Check sheet for the modelled part. Datum: model origin and axes. Units: mm. A direction names the side the tool comes from. Round coordinates to 2 decimals unless told otherwise and drop trailing zeros. Order: outer loops, then holes, each group sorted by start corner. A loop starts at its lowest first (then second) coordinate and runs counter-clockwise, first axis right, second up. Notation, with made-up numbers: (48, 74) -> (100, 74) arc R11 ccw to (100, 79) -> close; hole circle Ø4 at (56, 72). An arc over 180 degrees is marked (long way). Answer in a Markdown table with one row per item. Add a question column.
1. Access from +Z, -Z, +X, -X, +Y, -Y to the whole of each face (thin tool, end or side, straight path). Record for faces 4 (the cylindrical face through (3.34, 0.99, -0.37)), 5 (the flat face through (0, 7, -12.375)), 6 (the flat face through (15.798, 1.014, 7.113)), 7 (the flat face through (15, 2, 2)).
2. Depth check by flat-ended pin: P1, Ø4.5, axis at x = -5, z = 0, coming from the +Y side; P2, Ø6, axis at x = 15.5, z = -1.5, coming from the +Y side; P3, Ø3.5, axis at x = -16.75, z = -9.375, coming from the -Y side. Enter the tip coordinate at first touch or a pass-through.
3. Draft check along X on faces 1 (the flat face through (13.108, 1.014, 6.878)), 2 (the flat face through (0, 4.5, 0)), 3 (the flat face through (-22.75, 3, 0)). Enter one of: +X half, -X half, draft (parallel to the pull), parting line (faces both ways), or undercut.
4. Sectioned sample at C-C, the plane x = 15. Record the boundary of the cut face in (y, z) (3 decimals).
5. Sectioned sample at B-B, the plane x = -5. Record the boundary of the cut face in (y, z) (3 decimals), then the cut area to 3 significant figures.
6. Material ranges on L1, parallel to Z at x = 18, y = 5.5 (3 decimals); L2, parallel to Z at x = -16, y = 2.75 (3 decimals); L3, parallel to Z at x = 5, y = 3.4 (3 decimals), recorded low to high. Write a range as from..to.
7. Sectioned sample at A-A, the plane y = 6. Record the boundary of the cut face in (x, z) (3 decimals).
8. Sectioned sample at D-D, the plane z = 8.5. Record the boundary of the cut face in (x, y), then the cut area to 3 significant figures.
```python
from build123d import *

# Parameters (mm, degrees)
SKETCH1_W           = 45.5
SKETCH1_H           = 28.75
SKETCH1_R           = 1.7
BOSS_EXTRUDE1_DEPTH = 2
BOSS_EXTRUDE2_DEPTH = 7
SKETCH3_W           = 45.5
SKETCH3_H           = 8
SKETCH3_R           = 1.425
SKETCH3_R_2         = 1.685028189
BOSS_EXTRUDE3_DEPTH = 2.5
CUT_EXTRUDE1_REACH  = 29.807


with BuildPart() as part:
    # Sketch1 → Boss-Extrude1 (new body)
    with BuildSketch(Plane(origin=(0, 0, 0), x_dir=(1, 0, 0), z_dir=(0, 1, 0))):
        Rectangle(SKETCH1_W, SKETCH1_H)
        with Locations(Location((-15, 0, 0), (0, 0, 270))):
            Circle(SKETCH1_R, mode=Mode.SUBTRACT)
        with Locations(Location((-5, 0, 0), (0, 0, 270))):
            Circle(SKETCH1_R, mode=Mode.SUBTRACT)
        with Locations(Location((5, 0, 0), (0, 0, 270))):
            Circle(SKETCH1_R, mode=Mode.SUBTRACT)
        with Locations(Location((15, 0, 0), (0, 0, 270))):
            Circle(SKETCH1_R, mode=Mode.SUBTRACT)
    extrude(amount=BOSS_EXTRUDE1_DEPTH)

    # Sketch2 → Boss-Extrude2 (add)
    with BuildSketch(Plane(origin=(0, 2, 0), x_dir=(1, 0, 0), z_dir=(0, 1, 0))):
        Polygon((-22.75, 14.375), (22.75, 14.375), (22.75, 12.375), (20.75, 12.375), (-20.75, 12.375), (-22.75, 12.375), align=None)
        Polygon((-22.75, -14.375), (22.75, -14.375), (22.75, -12.375), (20.75, -12.375), (-20.75, -12.375), (-22.75, -12.375), align=None)
    extrude(amount=BOSS_EXTRUDE2_DEPTH)

    # Sketch3 → Boss-Extrude3 (add)
    # profile 1 of 4: a face of its own
    with BuildSketch(Plane(origin=(0, 2, 0), x_dir=(1, 0, 0), z_dir=(0, 1, 0))):
        with Locations((0, 8.375)):
            Rectangle(SKETCH3_W, SKETCH3_H)
        with Locations(Location((-16.75, 9.375, 0), (0, 0, 270))):
            Circle(SKETCH3_R, mode=Mode.SUBTRACT)
    # profile 2 of 4: a face of its own
    with BuildSketch(Plane(origin=(0, 2, 0), x_dir=(1, 0, 0), z_dir=(0, 1, 0))):
        with BuildLine():
            Line((22.75, 4.375), (-22.75, 4.375))
            Line((-22.75, 4.375), (-22.75, 0))
            Line((-22.75, 0), (-17.75, 0))
            ThreePointArc((-17.75, 0), (-15, 2.75), (-12.25, 0))
            Line((-12.25, 0), (-7.75, 0))
            ThreePointArc((-7.75, 0), (-5, 2.75), (-2.25, 0))
            Line((-2.25, 0), (2.25, 0))
            ThreePointArc((2.25, 0), (5, 2.75), (7.75, 0))
            Line((7.75, 0), (12.25, 0))
            ThreePointArc((12.25, 0), (15, 2.75), (17.75, 0))
            Line((17.75, 0), (22.75, 0))
            Line((22.75, 0), (22.75, 4.375))
        make_face()
    # profile 3 of 4: a face of its own
    with BuildSketch(Plane(origin=(0, 2, 0), x_dir=(1, 0, 0), z_dir=(0, 1, 0))):
        with BuildLine():
            Line((-17.75, 0), (-22.75, 0))
            Line((-22.75, 0), (-22.75, -4.375))
            Line((-22.75, -4.375), (22.75, -4.375))
            Line((22.75, -4.375), (22.75, 0))
            Line((22.75, 0), (17.75, 0))
            ThreePointArc((17.75, 0), (15, -2.75), (12.25, 0))
            Line((12.25, 0), (7.75, 0))
            ThreePointArc((7.75, 0), (5, -2.75), (2.25, 0))
            Line((2.25, 0), (-2.25, 0))
            ThreePointArc((-2.25, 0), (-5, -2.75), (-7.75, 0))
            Line((-7.75, 0), (-12.25, 0))
            ThreePointArc((-12.25, 0), (-15, -2.75), (-17.75, 0))
        make_face()
    # profile 4 of 4: a face of its own
    with BuildSketch(Plane(origin=(0, 2, 0), x_dir=(1, 0, 0), z_dir=(0, 1, 0))):
        with Locations((0, -8.375)):
            Rectangle(SKETCH3_W, SKETCH3_H)
        with Locations(Location((14.25, -9.325, 0), (0, 0, 270))):
            Circle(SKETCH3_R_2, mode=Mode.SUBTRACT)
    extrude(amount=BOSS_EXTRUDE3_DEPTH)

    # Sketch4 → Cut-Extrude1 (cut, up to next)
    with BuildSketch(Plane(origin=(0, 2, 0), x_dir=(1, 0, 0), z_dir=(0, 1, 0)), mode=Mode.PRIVATE) as cut_extrude1_sk1:
        Polygon((-19.867691454, 9.375), (-18.308845727, 6.675), (-15.191154273, 6.675), (-13.632308546, 9.375), (-15.191154273, 12.075), (-18.308845727, 12.075), align=None)
    cut_extrude1_tool1 = extrude(cut_extrude1_sk1.sketch, amount=-CUT_EXTRUDE1_REACH, mode=Mode.PRIVATE) & part.part
    # Sketch4 → Cut-Extrude1 (cut, up to next)
    with BuildSketch(Plane(origin=(0, 2, 0), x_dir=(1, 0, 0), z_dir=(0, 1, 0)), mode=Mode.PRIVATE) as cut_extrude1_sk2:
        Polygon((14.495583037, -6.216995983), (11.681181084, -7.558316843), (11.435598047, -10.66632086), (14.004416963, -12.433004017), (16.818818916, -11.091683157), (17.064401953, -7.98367914), align=None)
    cut_extrude1_tool2 = extrude(cut_extrude1_sk2.sketch, amount=-CUT_EXTRUDE1_REACH, mode=Mode.PRIVATE) & part.part
    add(cut_extrude1_tool1.solids().sort_by_distance((-16.75, 2, -9.375))[0], mode=Mode.SUBTRACT)
    add(cut_extrude1_tool2.solids().sort_by_distance((14.25, 2, 9.325))[0], mode=Mode.SUBTRACT)


solid = part.part
```
Answer key:
| question | item | result |
|---|---|---|
| 1 | face 4 | +Y, -Y |
| 1 | face 5 | +X, -X, +Y |
| 1 | face 6 | -Y |
| 1 | face 7 | +Y |
| 2 | P1 | stops at y = 2 |
| 2 | P2 | stops at y = 4.5 |
| 2 | P3 | stops at y = 2 |
| 3 | face 1 | undercut |
| 3 | face 2 | draft |
| 3 | face 3 | -X half |
| 4 | outline | (0, -14.375) -> (9, -14.375) -> (9, -12.375) -> (4.5, -12.375) -> (4.5, -2.75) -> (2, -2.75) -> (2, -1.7) -> (0, -1.7) -> close; (0, 1.7) -> (2, 1.7) -> (2, 2.75) -> (4.5, 2.75) -> (4.5, 7.816) -> (2, 7.816) -> (2, 6.564) -> (0, 6.564) -> close; (0, 11.959) -> (2, 11.959) -> (2, 10.834) -> (4.5, 10.834) -> (4.5, 12.375) -> (9, 12.375) -> (9, 14.375) -> (0, 14.375) -> close |
| 5 | outline | (0, -14.375) -> (9, -14.375) -> (9, -12.375) -> (4.5, -12.375) -> (4.5, -2.75) -> (2, -2.75) -> (2, -1.7) -> (0, -1.7) -> close; (0, 1.7) -> (2, 1.7) -> (2, 2.75) -> (4.5, 2.75) -> (4.5, 12.375) -> (9, 12.375) -> (9, 14.375) -> (0, 14.375) -> close |
| 5 | area | 127 mm² |
| 6 | L1 | z = -14.375..-12.375, 12.375..14.375 |
| 6 | L2 | z = -14.375..-10.587, -8.163..-2.562, 2.562..14.375 |
| 6 | L3 | z = -14.375..-2.75, 2.75..14.375 |
| 7 | outline | (-22.75, -14.375) -> (22.75, -14.375) -> (22.75, -12.375) -> (-22.75, -12.375) -> close; (-22.75, 12.375) -> (22.75, 12.375) -> (22.75, 14.375) -> (-22.75, 14.375) -> close |
| 8 | outline | (-22.75, 0) -> (11.61, 0) -> (11.61, 2) -> (12.78, 2) -> (12.78, 4.5) -> (-22.75, 4.5) -> close; (15.72, 2) -> (17.02, 2) -> (17.02, 0) -> (22.75, 0) -> (22.75, 4.5) -> (15.72, 4.5) -> close |
| 8 | area | 187 mm² |
